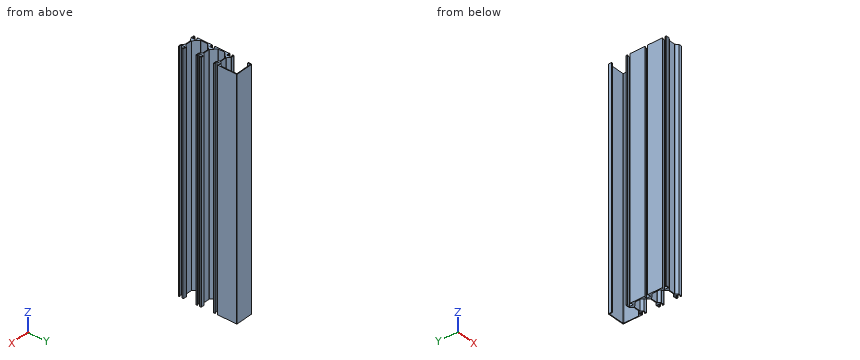
```python
from build123d import *

# Parameters (mm, degrees)
F1_DEPTH = 1000


with BuildPart() as f1:
    # F0 (on Top) → F1 (new body)
    with BuildSketch(Plane.XY):
        with BuildLine():
            Line((0, 8.917465), (0, 3.75))
            Line((0, 3.75), (3, 3.75))
            Line((3, 3.75), (3, 7))
            Line((3, 7), (13, 7))
            Line((13, 7), (13, -10))
            Line((13, -10), (3, -10))
            Line((3, -10), (3, -6.75))
            Line((3, -6.75), (0, -6.75))
            Line((0, -6.75), (0, -70.421975))
            Line((0, -70.421975), (3, -70.421975))
            Line((3, -70.421975), (3, -67.171975))
            Line((3, -67.171975), (13, -67.171975))
            Line((13, -67.171975), (13, -84.171975))
            Line((13, -84.171975), (3, -84.171975))
            Line((3, -84.171975), (3, -80.921975))
            Line((3, -80.921975), (0, -80.921975))
            Line((0, -80.921975), (0, -146.421568))
            Line((0, -146.421568), (3, -146.421568))
            Line((3, -146.421568), (3, -143.171568))
            Line((3, -143.171568), (13, -143.171568))
            Line((13, -143.171568), (13, -160.171568))
            Line((13, -160.171568), (3, -160.171568))
            Line((3, -160.171568), (3, -156.921568))
            Line((3, -156.921568), (0, -156.921568))
            Line((0, -156.921568), (0, -161.171568))
            ThreePointArc((0, -161.171568), (0.585786, -162.585782), (2, -163.171568))
            Line((2, -163.171568), (14.213203, -163.171568))
            Line((14.213203, -163.171568), (26.213203, -153.171568))
            Line((26.213203, -153.171568), (52.958573, -153.171568))
            ThreePointArc((52.958573, -153.171568), (53.72394, -153.323809), (54.372786, -153.757355))
            Line((54.372786, -153.757355), (63.201214, -162.585782))
            ThreePointArc((63.201214, -162.585782), (63.85006, -163.019327), (64.615427, -163.171568))
            Line((64.615427, -163.171568), (76, -163.171568))
            ThreePointArc((76, -163.171568), (77.414214, -162.585782), (78, -161.171568))
            Line((78, -161.171568), (78, -156.921568))
            Line((78, -156.921568), (75, -156.921568))
            Line((75, -156.921568), (75, -160.171568))
            Line((75, -160.171568), (65, -160.171568))
            Line((65, -160.171568), (65, -143.171568))
            Line((65, -143.171568), (75, -143.171568))
            Line((75, -143.171568), (75, -146.421568))
            Line((75, -146.421568), (78, -146.421568))
            Line((78, -146.421568), (78, -142.171568))
            ThreePointArc((78, -142.171568), (77.414214, -140.757355), (76, -140.171568))
            Line((76, -140.171568), (64.615427, -140.171568))
            ThreePointArc((64.615427, -140.171568), (63.85006, -140.323809), (63.201214, -140.757355))
            Line((63.201214, -140.757355), (54.372786, -149.585782))
            ThreePointArc((54.372786, -149.585782), (53.72394, -150.019327), (52.958573, -150.171568))
            Line((52.958573, -150.171568), (27.041631, -150.171568))
            ThreePointArc((27.041631, -150.171568), (26.276264, -150.019327), (25.627417, -149.585782))
            Line((25.627417, -149.585782), (5.585786, -129.544151))
            ThreePointArc((5.585786, -129.544151), (5.152241, -128.895305), (5, -128.129938))
            Line((5, -128.129938), (5, -99.213743))
            ThreePointArc((5, -99.213743), (5.152241, -98.448376), (5.585786, -97.79953))
            Line((5.585786, -97.79953), (26.203506, -77.18181))
            ThreePointArc((26.203506, -77.18181), (26.208346, -77.176986), (26.213203, -77.172179))
            Line((26.213203, -77.172179), (52.958776, -77.172179))
            ThreePointArc((52.958776, -77.172179), (53.724143, -77.32442), (54.37299, -77.757965))
            Line((54.37299, -77.757965), (63.201214, -86.586189))
            ThreePointArc((63.201214, -86.586189), (63.85006, -87.019734), (64.615427, -87.171975))
            Line((64.615427, -87.171975), (76, -87.171975))
            ThreePointArc((76, -87.171975), (77.414214, -86.586189), (78, -85.171975))
            Line((78, -85.171975), (78, -80.921975))
            Line((78, -80.921975), (75, -80.921975))
            Line((75, -80.921975), (75, -84.171975))
            Line((75, -84.171975), (65, -84.171975))
            Line((65, -84.171975), (65, -67.171975))
            Line((65, -67.171975), (75, -67.171975))
            Line((75, -67.171975), (75, -72.212282))
            Line((75, -72.212282), (78, -72.212282))
            Line((78, -72.212282), (78, -66.171975))
            ThreePointArc((78, -66.171975), (77.414214, -64.757762), (76, -64.171975))
            Line((76, -64.171975), (64.615427, -64.171975))
            ThreePointArc((64.615427, -64.171975), (63.85006, -64.324216), (63.201214, -64.757762))
            Line((63.201214, -64.757762), (54.37299, -73.585985))
            ThreePointArc((54.37299, -73.585985), (53.724143, -74.019531), (52.958776, -74.171772))
            Line((52.958776, -74.171772), (27.462442, -74.171772))
            ThreePointArc((27.462442, -74.171772), (26.485926, -74.127537), (25.647012, -73.625777))
            Line((25.647012, -73.625777), (5.585068, -53.543433))
            ThreePointArc((5.585068, -53.543433), (5.152047, -52.894835), (5, -52.129938))
            Line((5, -52.129938), (5, -26.213199))
            ThreePointArc((5, -26.213199), (5.152241, -25.447832), (5.585786, -24.798985))
            Line((5.585786, -24.798985), (26.213203, -4.171772))
            Line((26.213203, -4.171772), (53.787203, -4.171772))
            Line((53.787203, -4.171772), (62.615432, -13))
            Line((62.615432, -13), (76, -13))
            Line((76, -13), (76, -6.75))
            Line((76, -6.75), (73, -6.75))
            Line((73, -6.75), (73, -10))
            Line((73, -10), (63, -10))
            Line((63, -10), (63, 7))
            Line((63, 7), (73, 7))
            Line((73, 7), (73, 4.045606))
            Line((73, 4.045606), (76, 4.045606))
            Line((76, 4.045606), (76, 84.828228))
            ThreePointArc((76, 84.828228), (75.414214, 86.242442), (74, 86.828228))
            Line((74, 86.828228), (2, 86.828228))
            ThreePointArc((2, 86.828228), (0.585786, 86.242442), (0, 84.828228))
            Line((0, 84.828228), (0, 71.828228))
            Line((0, 71.828228), (3, 71.828228))
            Line((3, 71.828228), (3, 81.828228))
            ThreePointArc((3, 81.828228), (3.585786, 83.242442), (5, 83.828228))
            Line((5, 83.828228), (71, 83.828228))
            ThreePointArc((71, 83.828228), (72.414214, 83.242442), (73, 81.828228))
            Line((73, 81.828228), (73, 18.869452))
            ThreePointArc((73, 18.869452), (72.847759, 18.104085), (72.414214, 17.455238))
            Line((72.414214, 17.455238), (54.37299, -0.585985))
            ThreePointArc((54.37299, -0.585985), (53.724143, -1.019531), (52.958776, -1.171772))
            Line((52.958776, -1.171772), (27.041631, -1.171772))
            ThreePointArc((27.041631, -1.171772), (26.276264, -1.019531), (25.627417, -0.585985))
            Line((25.627417, -0.585985), (14.709753, 10.331678))
            ThreePointArc((14.709753, 10.331678), (14.060907, 10.765224), (13.29554, 10.917465))
            Line((13.29554, 10.917465), (2, 10.917465))
            ThreePointArc((2, 10.917465), (0.585786, 10.331678), (0, 8.917465))
        make_face()
    extrude(amount=F1_DEPTH)


solid = f1.part
```
Can you work these out from the model? Positions are in its coordinate system, mm. Coordinates: 2 decimals unless noted, no trailing zeros. Order: outer loops, then holes, each group sorted by start corner. A loop starts at its lowest first (then second) coordinate and runs counter-clockwise, first axis right, second up.
1. I'm going to push flat-ended pins straight in: pin 1 (1.5 mm diameter, centred on x = 20.5, z = 283, fed in from -Y); pin 2 (0.9 mm diameter, centred on x = 76, z = 719.5, fed in from +Y); pin 3 (3 mm diameter, centred on y = -24.5, z = 184.5, fed in from +X); pin 4 (2 mm diameter, centred on x = 31, y = 1, fed in from +Z). Where does each tip first touch, or does it pass through?
2. If we section it at A-A (x = 43): Please give me the cut outline in (y, z), then the cut area to 3 significant figures.
3. If we section it at B-B (y = 43): Please give me the cut outline in (x, z).
4. I need wall thicknesses on line 1 (Y direction, x = 46, z = 78.5); line 2 (X direction, y = -68.5, z = 147); line 3 (Y direction, x = 17.5, z = 188.5). Which ranges of each line are inside material? Lowest first, please.
Entries:
1. pin 1: stops at y = -158.56
1. pin 2: stops at y = 86.09
1. pin 3: stops at x = 7.38
1. pin 4: passes through
2. outline: (-153.17, 0) - (-150.17, 0) - (-150.17, 1000) - (-153.17, 1000) - close; (-77.17, 0) - (-74.17, 0) - (-74.17, 1000) - (-77.17, 1000) - close; (-4.17, 0) - (-1.17, 0) - (-1.17, 1000) - (-4.17, 1000) - close; (83.83, 0) - (86.83, 0) - (86.83, 1000) - (83.83, 1000) - close
2. area: 12,000 mm2
3. outline: (73, 0) - (76, 0) - (76, 1000) - (73, 1000) - close
4. line 1: y = -153.17 to -150.17, -77.17 to -74.17, -4.17 to -1.17, 83.83 to 86.83
4. line 2: x = 0 to 3, 13 to 20.53, 59.46 to 65, 75 to 78
4. line 3: y = -160.43 to -141.46, -85.89 to -65.47, -12.88 to 7.54, 83.83 to 86.83
